Drawing for the job (mm, zero at the part's lowest x, y, z). A direction names the side the tool comes from. Give positions to 0.01 mm unless a question says otherwise; leave off trailing zeros. Loops run counter-clockwise (first coordinate to the right, second up) from the corner with the lowest first, then second, coordinate; pieces in that order, holes last.
1) Flat gauge pins, fed straight in: P1, Ø3, axis at x = 21, y = 18, coming from the -Z side; P2, Ø5, axis at x = 3, y = 13, coming from the +Z side; P3, Ø7.5, axis at x = 13.5, y = 5, coming from the +Z side; P4, Ø8, axis at x = 15, z = 19, coming from the -Y side. Where does each tip first touch, or does it go through?
2) Band-saw the part on D-D on z = 22.5. List the corners of the cut face in (x, y).
3) Band-saw the part on C-C on z = 15.75. List the corners of the cut face in (x, y), then the cut area to 3 significant figures.
4) Wall check: line 1 (Z direction, x = 8.25, y = 17.5); line 2 (Z direction, x = 24.5, y = 4); line 3 (X direction, y = 11, z = 12.75). Give the ranges that are in metal, low to high.
5) Band-saw the part on A-A on y = 5.25. List the corners of the cut face in (x, z).
6) Band-saw the part on B-B on x = 20.5. List the corners of the cut face in (y, z), then the cut area to 3 significant figures.
7) Two-plate mould, pull along X, no slides. Class the marked faces 1, 2, 3 and 4: +X half, -X half, draft (parallel to the pull), parting line (faces both ways), or undercut.
8) 3-axis set-ups, long thin cutter, end or side, ignore diameter. For the marked faces 5, 6, 7 and 8: which of +Z, -Z, +X, -X, +Y, -Y reach the whole face in a straight line?
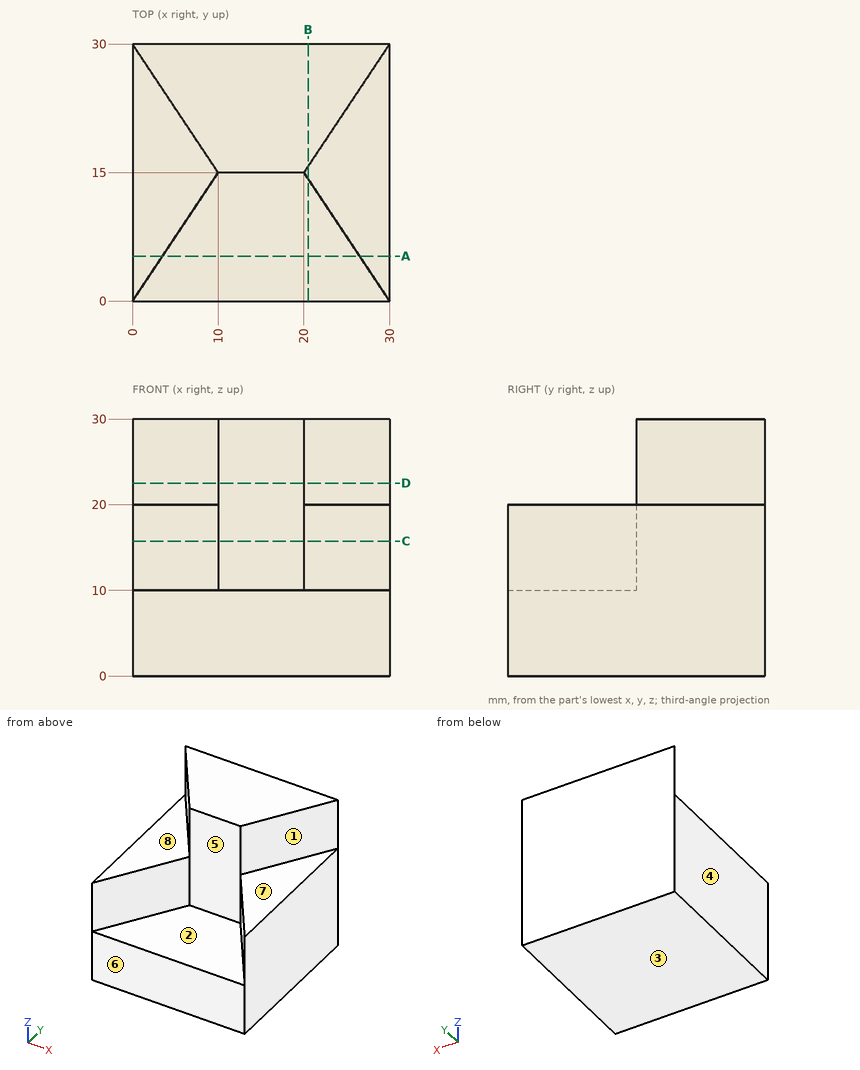
Findings below:
1. P1: stops at z = 0
1. P2: stops at z = 20
1. P3: stops at z = 10
1. P4: stops at y = 15
2. outline: (0, 30) - (10, 15) - (20, 15) - (30, 30) - close
3. outline: (0, 0) - (10, 15) - (20, 15) - (30, 0) - (30, 30) - (0, 30) - close
3. area: 600 mm2
4. line 1: z = 0 to 20
4. line 2: z = 0 to 10
4. line 3: x = 0 to 7.33, 22.67 to 30
5. outline: (0, 0) - (30, 0) - (30, 20) - (26.5, 20) - (26.5, 10) - (3.5, 10) - (3.5, 20) - (0, 20) - close
6. outline: (0, 0) - (30, 0) - (30, 30) - (15.75, 30) - (15.75, 20) - (14.25, 20) - (14.25, 10) - (0, 10) - close
6. area: 600 mm2
7. face 1: +X half
7. face 2: undercut
7. face 3: draft
7. face 4: -X half
8. face 5: +Z, -Y
8. face 6: +Z, -Z, +X, -X, -Y
8. face 7: +Z, +X, -Y
8. face 8: +Z, -X, -Y
